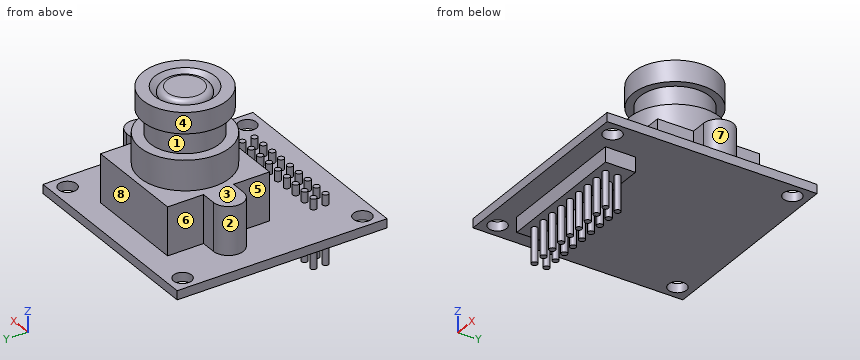
from build123d import *

# Parameters (mm, degrees)
CROQUIS1_W              = 34
CROQUIS1_H              = 35
CROQUIS1_R              = 1.5
SALIENTE_EXTRUIR1_DEPTH = 1.5
CROQUIS2_W              = 22.5
CROQUIS2_H              = 5
SALIENTE_EXTRUIR2_DEPTH = 2.5
SALIENTE_EXTRUIR3_DEPTH = 8
CROQUIS4_R              = 7.5
SALIENTE_EXTRUIR4_DEPTH = 5
CROQUIS5_R              = 5.75
SALIENTE_EXTRUIR5_DEPTH = 4
CROQUIS6_R              = 7
SALIENTE_EXTRUIR6_DEPTH = 3.5
CROQUIS7_R              = 5
CORTAR_EXTRUIR1_DEPTH   = 1
CORTAR_EXTRUIR1_DRAFT   = -45
CROQUIS8_R              = 4
SALIENTE_EXTRUIR7_DEPTH = 1
REDONDEO1_R             = 1
CROQUIS10_R             = 0.5
SALIENTE_EXTRUIR8_DEPTH = 5.75


with BuildPart() as part:
    # Croquis1 → Saliente-Extruir1 (new body)
    with BuildSketch(Plane.XY):
        Rectangle(CROQUIS1_W, CROQUIS1_H)
        with Locations((-14.571428571, 15)):
            Circle(CROQUIS1_R, mode=Mode.SUBTRACT)
        with Locations(Location((14.571428571, 15, 0), (0, 0, 180))):
            Circle(CROQUIS1_R, mode=Mode.SUBTRACT)
        with Locations((14.571428571, -15)):
            Circle(CROQUIS1_R, mode=Mode.SUBTRACT)
        with Locations(Location((-14.571428571, -15, 0), (0, 0, 180))):
            Circle(CROQUIS1_R, mode=Mode.SUBTRACT)
    extrude(amount=SALIENTE_EXTRUIR1_DEPTH)

    # Croquis2 → Saliente-Extruir2 (add)
    with BuildSketch(Plane(origin=(0, 0, 0), x_dir=(-1, 0, 0), z_dir=(0, 0, -1))):
        with Locations((0, -11.5)):
            Rectangle(CROQUIS2_W, CROQUIS2_H)
    extrude(amount=SALIENTE_EXTRUIR2_DEPTH)

    # Croquis3 → Saliente-Extruir3 (add)
    with BuildSketch(Plane.XY.offset(1.5)):
        with BuildLine():
            Line((-8.5, 13.5), (8.5, 13.5))
            Line((8.5, 13.5), (8.5, 7.5))
            Line((8.5, 7.5), (11, 7.5))
            ThreePointArc((11, 7.5), (13.5, 5), (11, 2.5))
            Line((11, 2.5), (8.5, 2.5))
            Line((8.5, 2.5), (8.5, -3.5))
            Line((8.5, -3.5), (-8.5, -3.5))
            Line((-8.5, -3.5), (-8.5, 2.5))
            Line((-8.5, 2.5), (-11, 2.5))
            ThreePointArc((-11, 2.5), (-13.5, 5), (-11, 7.5))
            Line((-11, 7.5), (-8.5, 7.5))
            Line((-8.5, 7.5), (-8.5, 13.5))
        make_face()
    extrude(amount=SALIENTE_EXTRUIR3_DEPTH)

    # Croquis4 → Saliente-Extruir4 (add)
    with BuildSketch(Plane.XY.offset(9.5)):
        with Locations((0, 5)):
            Circle(CROQUIS4_R)
    extrude(amount=SALIENTE_EXTRUIR4_DEPTH)

    # Croquis5 → Saliente-Extruir5 (add)
    with BuildSketch(Plane.XY.offset(14.5)):
        with Locations((0, 5)):
            Circle(CROQUIS5_R)
    extrude(amount=SALIENTE_EXTRUIR5_DEPTH)

    # Croquis6 → Saliente-Extruir6 (add)
    with BuildSketch(Plane.XY.offset(18.5)):
        with Locations(Location((0, 5, 0), (0, 0, 180))):
            Circle(CROQUIS6_R)
    extrude(amount=SALIENTE_EXTRUIR6_DEPTH)


with BuildPart() as cortar_extruir1_tool:
    # Croquis7 → Cortar-Extruir1 (with draft: the straight prism first)
    with BuildSketch(Plane.XY.offset(22)):
        with Locations((0, 5)):
            Circle(CROQUIS7_R)
    extrude(amount=-CORTAR_EXTRUIR1_DEPTH)
    # Cortar-Extruir1: the draft: its side faces are tilted about the plane it starts from
    cortar_extruir1_sides = [cortar_extruir1_tool.faces().sort_by_distance(p)[0] for p in [
        (-5, 5, 21.5),
    ]]
    draft(cortar_extruir1_sides, Plane.XY.offset(22), CORTAR_EXTRUIR1_DRAFT)


with BuildPart() as part_1:
    add(part.part)

    # Cortar-Extruir1: cut by cortar_extruir1_tool
    add(cortar_extruir1_tool.part, mode=Mode.SUBTRACT)

    # Croquis8 → Saliente-Extruir7 (add)
    with BuildSketch(Plane.XY.offset(21)):
        with Locations((0, 5)):
            Circle(CROQUIS8_R)
    extrude(amount=SALIENTE_EXTRUIR7_DEPTH)

    # Redondeo1
    redondeo1_edges = [part_1.edges().sort_by_distance(p)[0] for p in [
        (-4, 5, 22),
    ]]
    fillet(redondeo1_edges, radius=REDONDEO1_R - 0.0001)  # a hair under: the kernel refuses the full size

    # Croquis10 → Saliente-Extruir8 (add, symmetric)
    with BuildSketch(Plane(origin=(0, 0, -2.5), x_dir=(-1, 0, 0), z_dir=(0, 0, -1))):
        with Locations((-9, -12.5)):
            Circle(CROQUIS10_R)
        with Locations((-9, -10.5)):
            Circle(CROQUIS10_R)
        with Locations((-6.75, -10.5)):
            Circle(CROQUIS10_R)
        with Locations((-4.5, -10.5)):
            Circle(CROQUIS10_R)
        with Locations((-2.25, -10.5)):
            Circle(CROQUIS10_R)
        with Locations((0, -10.5)):
            Circle(CROQUIS10_R)
        with Locations((2.25, -10.5)):
            Circle(CROQUIS10_R)
        with Locations((4.5, -10.5)):
            Circle(CROQUIS10_R)
        with Locations((6.75, -10.5)):
            Circle(CROQUIS10_R)
        with Locations((9, -10.5)):
            Circle(CROQUIS10_R)
        with Locations((-6.75, -12.5)):
            Circle(CROQUIS10_R)
        with Locations((-4.5, -12.5)):
            Circle(CROQUIS10_R)
        with Locations((-2.25, -12.5)):
            Circle(CROQUIS10_R)
        with Locations((0, -12.5)):
            Circle(CROQUIS10_R)
        with Locations((2.25, -12.5)):
            Circle(CROQUIS10_R)
        with Locations((4.5, -12.5)):
            Circle(CROQUIS10_R)
        with Locations((6.75, -12.5)):
            Circle(CROQUIS10_R)
        with Locations((9, -12.5)):
            Circle(CROQUIS10_R)
    extrude(amount=SALIENTE_EXTRUIR8_DEPTH, both=True)


solid = part_1.part
For this review, take the finished solid that the model builds, in its own axes (mm). Face numbers are marked on the shaded views. A direction names the side the tool comes from. Give positions to 0.01 mm unless a question says otherwise; leave off trailing zeros. Order: outer loops, then holes, each group sorted by start corner. A loop starts at its lowest first (then second) coordinate and runs counter-clockwise, first axis right, second up. Notation, with made-up numbers: (-37, 71.25) - (-21, 71.25) arc R9 cw to (-21, 77.25) - close; hole circle Ø10 at (0.25, 77). An arc over 180 degrees is marked (long way). Answer as a JSON object with one key per item and string values. Group by question number.
Item 1: Draft analysis for pull direction Z (two halves, no side actions). For the marked faces 1, 2 and 3, state which applies: pulls with the +Z half, pulls with the -Z half, needs draft (parallel to the pull), parting line crosses it, or undercut.
Item 2: Machinability: for the marked faces 4, 5, 6, 7 and 8, which of the approach directions +Z, -Z, +X, -X, +Y, -Y give a long, thin tool a straight path to every point of the face, cutting with its end or side? Answer none if there is none.
Item 3: Take a section at B-B on x = 10.5. Give the boundary of the cut face in (y, z), and give its area (3 significant figures).
Item 4: Take a section at A-A on y = -15. Give the boundary of the cut face in (x, z).
Item 5: Wall thickness on line 1 along Y through (x, z) = (-1, -0.5); line 2 along Z through (x, y) = (-2.5, -4); line 3 along Y through (x, z) = (-11, 2): over which ranges is each line inside the solid? List them lowest first.
Item 6: Clearance check with flat-ended pins moving along their axes: pin 1 Ø5 at (y, z) = (10.5, 7) entering from -X; pin 2 Ø2 at (x, z) = (-10, 5.5) entering from -Y; pin 3 Ø4 at (y, z) = (6.5, 14.5) entering from -X. State where each tip first meets the part, or that it passes through.
Item 7: Take a section at D-D on x = 15. Give the boundary of the cut face in (y, z).
Item 8: Take a section at C-C on z = 5. Give the boundary of the cut face in (x, y).
Reported:
{
 "1": {"face 1": "undercut", "face 2": "needs draft", "face 3": "pulls with the +Z half"},
 "2": {"face 4": "+Z", "face 5": "+Z, -X", "face 6": "+Z, -X, +Y", "face 7": "+Z, +X", "face 8": "+Z, +X, -X, +Y"},
 "3": {"outline": "(-17.5, 0) - (-14, 0) - (-14, -2.5) - (-9, -2.5) - (-9, 0) - (17.5, 0) - (17.5, 1.5) - (7.5, 1.5) - (7.5, 9.5) - (2.5, 9.5) - (2.5, 1.5) - (-17.5, 1.5) - close", "area": "105 mm^2"},
 "4": {"outline": "(-17, 0) - (-16.07, 0) - (-16.07, 1.5) - (-17, 1.5) - close; (-13.07, 0) - (13.07, 0) - (13.07, 1.5) - (-13.07, 1.5) - close; (16.07, 0) - (17, 0) - (17, 1.5) - (16.07, 1.5) - close"},
 "5": {"line 1": "-14 to -9", "line 2": "0 to 1.5", "line 3": "2.5 to 7.5"},
 "6": {"pin 1": "x = -8.5", "pin 2": "y = 2.5", "pin 3": "x = -7.5"},
 "7": {"outline": "(-17.5, 0) - (-16.44, 0) - (-16.44, 1.5) - (-17.5, 1.5) - close; (-13.56, 0) - (13.56, 0) - (13.56, 1.5) - (-13.56, 1.5) - close; (16.44, 0) - (17.5, 0) - (17.5, 1.5) - (16.44, 1.5) - close"},
 "8": {"outline": "(-11, 2.5) - (-8.5, 2.5) - (-8.5, -3.5) - (8.5, -3.5) - (8.5, 2.5) - (11, 2.5) arc R2.5 ccw to (11, 7.5) - (8.5, 7.5) - (8.5, 13.5) - (-8.5, 13.5) - (-8.5, 7.5) - (-11, 7.5) arc R2.5 ccw to start"}
}
